For this review, use the dimensioned drawing (mm, ordinates from the lowest corner) and the shaded views. A direction names the side the tool comes from. Coordinates: 2 decimals unless noted, no trailing zeros. Order: outer loops, then holes, each group sorted by start corner. A loop starts at its lowest first (then second) coordinate and runs counter-clockwise, first axis right, second up. Notation, with made-up numbers: M -34,79 L -1,79 A35 cw -1,113 Z; hole C 56,14.5 d2. An arc over 180 degrees is marked long. One line per item, written item: value.
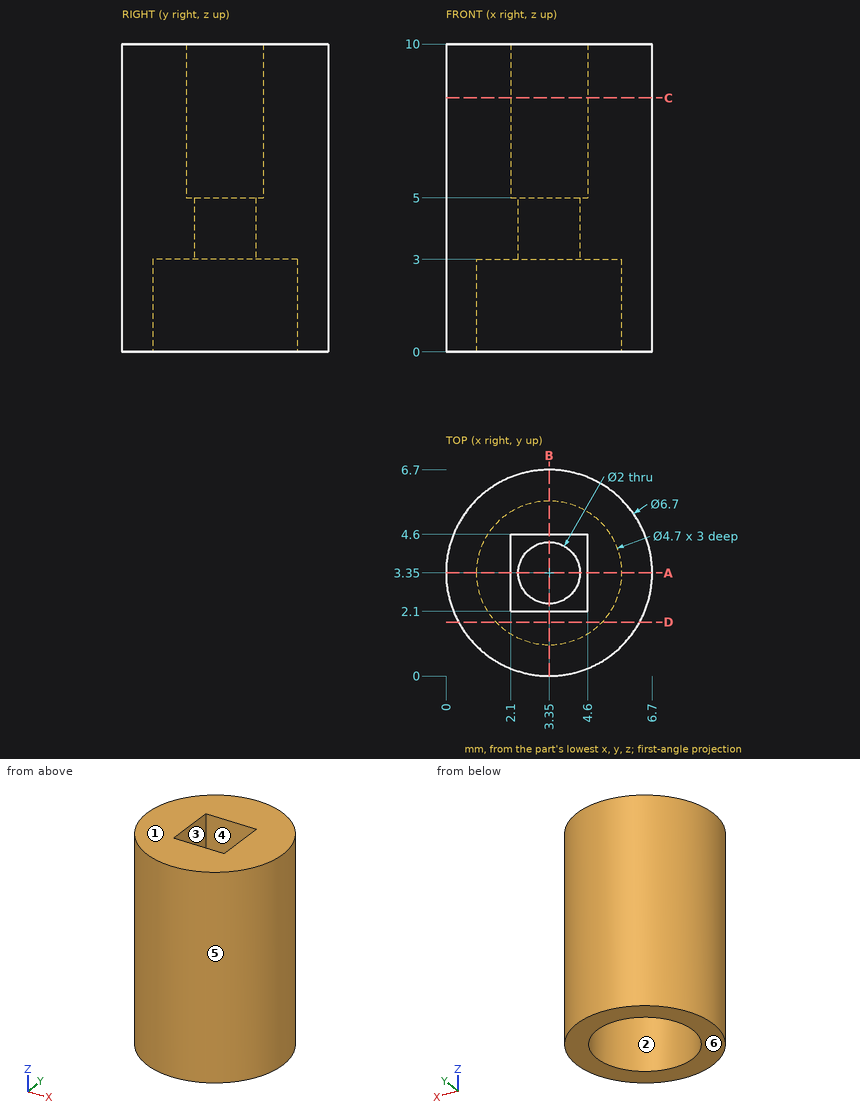
(1) Mouldability with a two-part tool opening along Y and no side actions: class the marked faces 3, 4, 5 and 6 as +Y half, -Y half, draft (parallel to the pull), parting line (faces both ways), or undercut.
Geometry results:
face 3: undercut
face 4: undercut
face 5: parting line
face 6: draft
(2) For L1, parallel to Y at x = 3.35, z = 3.45; L2, parallel to Y at x = 3.35, z = 2.25, list the stretches that pass through material, from the lowest coordinate up.
Geometry results:
L1: y = 0 to 2.35, 4.35 to 6.7
L2: y = 0 to 1, 5.7 to 6.7
(3) We need section C-C, the plane z = 8.25. State the section outline as (x, y) points, plus the area to 3 significant figures.
Geometry results:
outline: C 3.35,3.35 d6.7; hole M 2.1,2.1 L 4.6,2.1 L 4.6,4.6 L 2.1,4.6 Z
area: 29.0 mm2
(4) Tool access review of the marked faces 1 and 2: name each direction out of +Z, -Z, +X, -X, +Y, -Y from which nothing blocks a thin tool from reaching the whole face with its end or side.
Geometry results:
face 1: +Z, +X, -X, +Y, -Y
face 2: -Z
(5) We need section A-A, the plane y = 3.35. State the section outline as (x, z) points.
Geometry results:
outline: M 0,0 L 1,0 L 1,3 L 2.35,3 L 2.35,5 L 2.1,5 L 2.1,10 L 0,10 Z; M 4.35,3 L 5.7,3 L 5.7,0 L 6.7,0 L 6.7,10 L 4.6,10 L 4.6,5 L 4.35,5 Z
(6) Insertion check: pin 1 Ø2.5 at (x, y) = (3.35, 3.35) entering from -Z; pin 2 Ø1.2 at (y, z) = (3.5, 8) entering from -X; pin 3 Ø0.7 at (x, y) = (2.5, 3.5) entering from +Z; pin 4 Ø1 at (y, z) = (1.5, 6.5) entering from -X. Each pin has a flat end and moves straight along its axis. Give the tip position at first contact, or say it passes through.
Geometry results:
pin 1: stops at z = 3
pin 2: stops at x = 0
pin 3: stops at z = 5
pin 4: stops at x = 0.28
(7) We need section D-D, the plane y = 1.75. State the section outline as (x, z) points.
Geometry results:
outline: M 0.41,0 L 1.63,0 L 1.63,3 L 5.07,3 L 5.07,0 L 6.29,0 L 6.29,10 L 0.41,10 Z
